Design review of the part built by this model. Coordinates are the model's own, in mm. Give positions to 0.01 mm unless a question says otherwise; leave off trailing zeros. Write each loop counter-clockwise with the first axis right and the second up, starting at its lowest first coordinate (ties: lowest second). Pieces come first, ordered by that corner, then holes. Notation, with made-up numbers: (51.25, 34.5) -> (69.25, 34.5) arc R24 cw to (69.25, 53.5) -> close; hole circle Ø6 at (60, 13). An arc over 180 degrees is marked (long way). Put each result on its own line as item: value. Start each with the question number.
from build123d import *

# Parameters (mm, degrees)
BOSS_EXTRUDE1_DEPTH                        = 2
SKETCH6_R                                  = 1.5
CUT_EXTRUDE3_DEPTH                         = 4
MIRROR2_AT_THE_SECOND_PLANE_COPY_1_DEPTH   = 2
MIRROR2_AT_THE_SECOND_PLANE_COPY_2_SKETC_R = 1.5
MIRROR2_AT_THE_SECOND_PLANE_COPY_2_DEPTH   = 4


with BuildPart() as part:
    # Sketch1 → Boss-Extrude1 (new body)
    with BuildSketch(Plane(origin=(0, 0, 0), x_dir=(1, 0, 0), z_dir=(0, 1, 0))):
        Polygon((25, 40), (40, 25), (40, 0), (0, 0), (0, 40), align=None)
    boss_extrude1 = extrude(amount=BOSS_EXTRUDE1_DEPTH)

    # Sketch6 → Cut-Extrude3 (cut, through all)
    with BuildSketch(Plane(origin=(0, 3, 0), x_dir=(1, 0, 0), z_dir=(0, 1, 0))):
        with Locations((33, 24)):
            Circle(SKETCH6_R)
        with Locations((24, 33)):
            Circle(SKETCH6_R)
        with Locations((4, 33)):
            Circle(SKETCH6_R)
        with Locations((33, 4)):
            Circle(SKETCH6_R)
        with Locations((5, 5)):
            Circle(SKETCH6_R)
    cut_extrude3 = extrude(amount=-CUT_EXTRUDE3_DEPTH, mode=Mode.SUBTRACT)

    # Mirror2: Boss-Extrude1, Cut-Extrude3 across plane
    add(boss_extrude1.mirror(Plane(origin=(0, 0, 0), x_dir=(0, 0, 1), z_dir=(1, 0, 0))))
    add(cut_extrude3.mirror(Plane(origin=(0, 0, 0), x_dir=(0, 0, 1), z_dir=(1, 0, 0))), mode=Mode.SUBTRACT)

    # Mirror2 at the second plane: Boss-Extrude1, Cut-Extrude3 across plane
    add(boss_extrude1.mirror(Plane.XY))
    add(cut_extrude3.mirror(Plane.XY), mode=Mode.SUBTRACT)

    # Mirror2 at the second plane copy 1 sketc → Mirror2 at the second plane copy 1 (add)
    with BuildSketch(Plane(origin=(0, 0, 0), x_dir=(-1, 0, 0), z_dir=(0, 1, 0))):
        Polygon((25, 40), (40, 25), (40, 0), (0, 0), (0, 40), align=None)
    extrude(amount=MIRROR2_AT_THE_SECOND_PLANE_COPY_1_DEPTH)

    # Mirror2 at the second plane copy 2 sketc → Mirror2 at the second plane copy 2 (cut, through all)
    with BuildSketch(Plane(origin=(0, 3, 0), x_dir=(-1, 0, 0), z_dir=(0, 1, 0))):
        with Locations((33, 24)):
            Circle(MIRROR2_AT_THE_SECOND_PLANE_COPY_2_SKETC_R)
        with Locations((24, 33)):
            Circle(MIRROR2_AT_THE_SECOND_PLANE_COPY_2_SKETC_R)
        with Locations((4, 33)):
            Circle(MIRROR2_AT_THE_SECOND_PLANE_COPY_2_SKETC_R)
        with Locations((33, 4)):
            Circle(MIRROR2_AT_THE_SECOND_PLANE_COPY_2_SKETC_R)
        with Locations((5, 5)):
            Circle(MIRROR2_AT_THE_SECOND_PLANE_COPY_2_SKETC_R)
    extrude(amount=-MIRROR2_AT_THE_SECOND_PLANE_COPY_2_DEPTH, mode=Mode.SUBTRACT)


solid = part.part
Q1. For pin 1 (2.5 mm diameter, centred on x = -5, z = 5, fed in from +Y), flat-tipped, find the tip position at first contact; note if it passes through.
Q2. To check wall thickness, follow probe 1 along Z at (x, y) = (24, 0.25); probe 2 along Z at (x, y) = (4, 0.9); probe 3 along X at (y, z) = (0.7, 33.5). State the ranges of each line that lie inside material, in increasing order. Write a range as from..to.
Q3. Take a section at D-D on x = 33. Give the boundary of the cut face in (y, z), then the cut area to 3 significant figures.
Q4. Take a section at A-A on z = 24. Give the boundary of the cut face in (x, y), then the cut area to 3 significant figures.
Q5. Mouldability with a two-part tool opening along X and no side actions: class faces 1 (the face through (-40, 1, 0)), 2 (the face through (-4.69, 1.01, 31.67)), 3 (the face through (6.386, 1.014, 4.425)), 4 (the face through (32, 1, 33)) as +X half, -X half, draft (parallel to the pull), parting line (faces both ways), or undercut.
Q6. Take a section at C-C on y = 0.95. State how many separate pieces and enclosed holes the cut face has, then the cut area to 3 significant figures.
Q7. Take a section at B-B on x = -24. Give the boundary of the cut face in (y, z), then the cut area to 3 significant figures.
Result:
1. pin 1: passes through
2. probe 1: z = -40..-34.5, -31.5..31.5, 34.5..40
2. probe 2: z = -40..-34.5, -31.5..-6.12, -3.88..3.88, 6.12..31.5, 34.5..40
2. probe 3: x = -31.5..-25.41, -22.59..-5.41, -2.59..2.59, 5.41..22.59, 25.41..31.5
3. outline: (0, -32) -> (2, -32) -> (2, -25.5) -> (0, -25.5) -> close; (0, -22.5) -> (2, -22.5) -> (2, -5.5) -> (0, -5.5) -> close; (0, -2.5) -> (2, -2.5) -> (2, 2.5) -> (0, 2.5) -> close; (0, 5.5) -> (2, 5.5) -> (2, 22.5) -> (0, 22.5) -> close; (0, 25.5) -> (2, 25.5) -> (2, 32) -> (0, 32) -> close
3. area: 104 mm^2
4. outline: (-40, 0) -> (-34.5, 0) -> (-34.5, 2) -> (-40, 2) -> close; (-31.5, 0) -> (31.5, 0) -> (31.5, 2) -> (-31.5, 2) -> close; (34.5, 0) -> (40, 0) -> (40, 2) -> (34.5, 2) -> close
4. area: 148 mm^2
5. face 1: -X half
5. face 2: undercut
5. face 3: undercut
5. face 4: +X half
6. separate pieces: 1
6. enclosed holes: 20
6. area: 5,810 mm^2
7. outline: (0, -40) -> (2, -40) -> (2, -34.5) -> (0, -34.5) -> close; (0, -31.5) -> (2, -31.5) -> (2, 31.5) -> (0, 31.5) -> close; (0, 34.5) -> (2, 34.5) -> (2, 40) -> (0, 40) -> close
7. area: 148 mm^2
